```python
from build123d import *

# Parameters (mm, degrees)
SKETCH1_W               = 212.5
SKETCH1_H               = 339.725
BOSS_EXTRUDE1_DEPTH     = 6
SKETCH2_W               = 6.5
SKETCH2_H               = 20
BOSS_EXTRUDE2_DEPTH     = 24
CUT_EXTRUDE1_DEPTH      = 393.36344838
CUT_EXTRUDE1_DEPTH_BACK = 393.36344838
SKETCH3_R               = 4
FILLET2_R               = 5
SKETCH5_R               = 3.175
CUT_EXTRUDE2_DEPTH      = 402.314497153
CUT_EXTRUDE3_DEPTH      = 402.314497153
SKETCH10_R              = 4
CUT_EXTRUDE4_DEPTH      = 18
SKETCH11_R              = 4
CUT_EXTRUDE5_DEPTH      = 14.986


with BuildPart() as part:
    # Sketch1 → Boss-Extrude1 (new body)
    with BuildSketch(Plane.XY):
        with Locations((106.25, -169.8625)):
            Rectangle(SKETCH1_W, SKETCH1_H)
    extrude(amount=BOSS_EXTRUDE1_DEPTH)

    # Sketch2 → Boss-Extrude2 (add)
    with BuildSketch(Plane.XY.offset(6)):
        with Locations((21.75, -35.2425)):
            Rectangle(SKETCH2_W, SKETCH2_H)
        with Locations((50.75, -35.2425)):
            Rectangle(SKETCH2_W, SKETCH2_H)
        with Locations((190.75, -35.2425)):
            Rectangle(SKETCH2_W, SKETCH2_H)
        with Locations((161.75, -35.2425)):
            Rectangle(SKETCH2_W, SKETCH2_H)
        with Locations((133.75, -104.5325)):
            Rectangle(SKETCH2_W, SKETCH2_H)
        with Locations((165.25, -104.5325)):
            Rectangle(SKETCH2_W, SKETCH2_H)
        with Locations((165.25, -235.1925)):
            Rectangle(SKETCH2_W, SKETCH2_H)
        with Locations((21.75, -304.4825)):
            Rectangle(SKETCH2_W, SKETCH2_H)
        with Locations((50.75, -304.4825)):
            Rectangle(SKETCH2_W, SKETCH2_H)
        with Locations((190.75, -304.4825)):
            Rectangle(SKETCH2_W, SKETCH2_H)
        with Locations((161.75, -304.4825)):
            Rectangle(SKETCH2_W, SKETCH2_H)
        with Locations((133.75, -235.1925)):
            Rectangle(SKETCH2_W, SKETCH2_H)
    extrude(amount=BOSS_EXTRUDE2_DEPTH)

    # Sketch3 → Cut-Extrude1 (cut, two sides: drawn at the far end of the back side and taken through both)
    with BuildSketch(Plane.ZY.offset(-18.5).offset(-CUT_EXTRUDE1_DEPTH_BACK)):
        with Locations(Location((18, -35.2425, 0), (0, 0, 180))):
            Circle(SKETCH3_R)
        with Locations((18, -235.1925)):
            Circle(SKETCH3_R)
        with Locations(Location((18, -304.4825, 0), (0, 0, 270))):
            Circle(SKETCH3_R)
        with Locations(Location((18, -104.5325, 0), (0, 0, 180))):
            Circle(SKETCH3_R)
        with BuildLine():
            Line((18, -25.2425), (18, -12.982943413))
            Line((18, -12.982943413), (51.949532367, -12.982943413))
            Line((51.949532367, -12.982943413), (51.949532367, -57.481006387))
            Line((51.949532367, -57.481006387), (18, -57.481006387))
            Line((18, -57.481006387), (18, -45.2425))
            ThreePointArc((18, -45.2425), (28, -35.2425), (18, -25.2425))
        make_face()
        with BuildLine():
            Line((52.442304634, -132.399123951), (18, -132.399123951))
            Line((18, -132.399123951), (18, -114.5325))
            ThreePointArc((18, -114.5325), (28, -104.5325), (18, -94.5325))
            Line((18, -94.5325), (18, -71.59149594))
            Line((18, -71.59149594), (52.442304634, -71.59149594))
            Line((52.442304634, -71.59149594), (52.442304634, -132.399123951))
        make_face()
        with BuildLine():
            Line((52.599532243, -270.375386727), (18, -270.375386727))
            Line((18, -270.375386727), (18, -245.1925))
            ThreePointArc((18, -245.1925), (28, -235.1925), (18, -225.1925))
            Line((18, -225.1925), (18, -207.306351849))
            Line((18, -207.306351849), (52.599532243, -207.306351849))
            Line((52.599532243, -207.306351849), (52.599532243, -270.375386727))
        make_face()
        with BuildLine():
            Line((52.621034016, -326.721115515), (18, -326.721115515))
            Line((18, -326.721115515), (18, -314.4825))
            ThreePointArc((18, -314.4825), (28, -304.4825), (18, -294.4825))
            Line((18, -294.4825), (18, -282.222834285))
            Line((18, -282.222834285), (52.621034016, -282.222834285))
            Line((52.621034016, -282.222834285), (52.621034016, -326.721115515))
        make_face()
    extrude(amount=CUT_EXTRUDE1_DEPTH + CUT_EXTRUDE1_DEPTH_BACK, mode=Mode.SUBTRACT)

    # Fillet2
    fillet2_edges = [part.edges().sort_by_distance(p)[0] for p in [
        (190.75, -45.2425, 6),
        (194, -35.2425, 6),
        (190.75, -25.2425, 6),
        (50.75, -45.2425, 6),
        (54, -35.2425, 6),
        (50.75, -25.2425, 6),
        (21.75, -25.2425, 6),
        (18.5, -35.2425, 6),
        (21.75, -45.2425, 6),
        (161.75, -25.2425, 6),
        (158.5, -35.2425, 6),
        (161.75, -45.2425, 6),
        (161.75, -294.4825, 6),
        (161.75, -314.4825, 6),
        (158.5, -304.4825, 6),
        (190.75, -314.4825, 6),
        (194, -304.4825, 6),
        (190.75, -294.4825, 6),
        (165.25, -245.1925, 6),
        (168.5, -235.1925, 6),
        (165.25, -225.1925, 6),
        (133.75, -225.1925, 6),
        (130.5, -235.1925, 6),
        (133.75, -245.1925, 6),
        (50.75, -314.4825, 6),
        (54, -304.4825, 6),
        (50.75, -294.4825, 6),
        (21.75, -294.4825, 6),
        (21.75, -314.4825, 6),
        (18.5, -304.4825, 6),
        (165.25, -114.5325, 6),
        (165.25, -94.5325, 6),
        (168.5, -104.5325, 6),
        (133.75, -94.5325, 6),
        (130.5, -104.5325, 6),
        (133.75, -114.5325, 6),
    ]]
    fillet(fillet2_edges, radius=FILLET2_R)

    # Sketch5 → Cut-Extrude2 (cut, through all)
    with BuildSketch(Plane.XY.offset(6)):
        with Locations((12.7, -12.7)):
            Circle(SKETCH5_R)
        with Locations((199.8, -12.7)):
            Circle(SKETCH5_R)
        with Locations((66.25, -35.2425)):
            Circle(SKETCH5_R)
        with Locations((146.25, -35.2425)):
            Circle(SKETCH5_R)
        with Locations((176.25, -57.8625)):
            Circle(SKETCH5_R)
        with Locations((36.25, -57.8625)):
            Circle(SKETCH5_R)
        with Locations((191.25, -104.5325)):
            Circle(SKETCH5_R)
        with Locations((36.25, -169.8625)):
            Circle(SKETCH5_R)
        with Locations((191.25, -169.8625)):
            Circle(SKETCH5_R)
        with Locations((36.25, -281.8625)):
            Circle(SKETCH5_R)
        with Locations((66.25, -304.4825)):
            Circle(SKETCH5_R)
        with Locations((12.7, -327.025)):
            Circle(SKETCH5_R)
        with Locations((199.8, -327.025)):
            Circle(SKETCH5_R)
        with Locations((146.25, -304.4825)):
            Circle(SKETCH5_R)
        with Locations(Location((191.25, -235.1925, 0), (0, 0, 180))):
            Circle(SKETCH5_R)
    extrude(amount=-CUT_EXTRUDE2_DEPTH, mode=Mode.SUBTRACT)

    # Sketch9 → Cut-Extrude3 (cut, through all)
    with BuildSketch(Plane.XY.offset(6)):
        with BuildLine():
            Line((70, -271.3625), (110, -271.3625))
            ThreePointArc((110, -271.3625), (114.242640687, -269.605140687), (116, -265.3625))
            Line((116, -265.3625), (116, -74.3625))
            ThreePointArc((116, -74.3625), (114.242640687, -70.119859313), (110, -68.3625))
            Line((110, -68.3625), (70, -68.3625))
            ThreePointArc((70, -68.3625), (65.757359313, -70.119859313), (64, -74.3625))
            Line((64, -74.3625), (64, -265.3625))
            ThreePointArc((64, -265.3625), (65.757359313, -269.605140687), (70, -271.3625))
        make_face()
    extrude(amount=-CUT_EXTRUDE3_DEPTH, mode=Mode.SUBTRACT)

    # Sketch10 → Cut-Extrude4 (cut)
    with BuildSketch(Plane.XY.offset(6)):
        with Locations((76.95, -316.111459893)):
            Circle(SKETCH10_R)
    extrude(amount=-CUT_EXTRUDE4_DEPTH, mode=Mode.SUBTRACT)

    # Sketch11 → Cut-Extrude5 (cut)
    with BuildSketch(Plane.XY.offset(6)):
        with Locations((76.9625, -23.613540107)):
            Circle(SKETCH11_R)
    extrude(amount=-CUT_EXTRUDE5_DEPTH, mode=Mode.SUBTRACT)


solid = part.part
```
Read the model definition and answer for the solid it produces. Units are mm, in the model's axes. A direction names the side the tool comes from. Coordinates: 2 decimals unless noted, no trailing zeros. Write each loop counter-clockwise with the first axis right and the second up, starting at its lowest first coordinate (ties: lowest second). Pieces come first, ordered by that corner, then holes. Notation, with made-up numbers: (16, 83.25) -> (27, 83.25) arc R14 cw to (27, 96.25) -> close; hole circle Ø5 at (-4.5, 46). An arc over 180 degrees is marked (long way). Answer as a JSON object with one key per item and string values.
Q1. The part is cut by section B-B on y = -84. Give the vertices of the cut face in (x, z), then the cut area to 3 significant figures.
The answers:
{"outline": "(0, 0) -> (64, 0) -> (64, 6) -> (0, 6) -> close; (116, 0) -> (212.5, 0) -> (212.5, 6) -> (116, 6) -> close", "area": "963 mm2"}
Q2. Determine the mould class of faces 4 (the flat face through (54, -31, 19)), 5 (the cylindrical face through (78.81, -27.16, 3.04)), 6 (the flat face through (18.5, -31, 19)), 7 (the cylindrical face through (133.796, -239.097, 17.133)) for opening direction X: pulls with the +X half, pulls with the -X half, needs draft (parallel to the pull), parting line crosses it, or undercut.
The answers:
{"face 4": "undercut", "face 5": "undercut", "face 6": "pulls with the -X half", "face 7": "needs draft"}
Q3. The part is cut by section A-A on x = 87. Give the vertices of the cut face in (y, z) (1 decimal), then the cut area to 3 significant figures.
The answers:
{"outline": "(-339.7, 0) -> (-271.4, 0) -> (-271.4, 6) -> (-339.7, 6) -> close; (-68.4, 0) -> (0, 0) -> (0, 6) -> (-68.4, 6) -> close", "area": "820 mm2"}
Q4. Consider line 1 (Y direction, x = 199.8, z = 2.25) (3 decimals); line 2 (X direction, y = -35.5, z = 2); line 3 (X direction, y = -312.5, z = 22). Determine where each line is inside the solid, lowest interval first. Write a range as [from, to].
The answers:
{"line 1": "y = [-339.725, -330.2], [-323.85, -15.875], [-9.525, 0]", "line 2": "x = [0, 63.09], [69.41, 143.09], [149.41, 212.5]", "line 3": "x = [18.5, 25], [47.5, 54], [158.5, 165], [187.5, 194]"}
Q5. A tool of negligible diameter and unlimited length cuts with its end or side. For faces 1 (the flat face through (137, -101, 14)), 2 (the flat face through (51, -294.482, 14)), 3 (the flat face through (162, -101, 14)), from which of +Z, -Z, +X, -X, +Y, -Y can it reach the whole face along a straight path? Write none if from no direction.
The answers:
{"face 1": "+Z, +Y, -Y", "face 2": "+Z, +X, -X", "face 3": "+Z"}
Q6. Flat-ended cylindrical pins translate along their axes: pin 1 Ø7 at (x, z) = (22.5, 13) entering from +Y; pin 2 Ø3 at (x, z) = (160.5, 15) entering from -Y; pin 3 Ø7 at (x, z) = (164, 14.5) entering from +Y. Find the tip coordinate at first contact, or state that the pin passes through.
The answers:
{"pin 1": "stops at y = -25.01", "pin 2": "stops at y = -314.48", "pin 3": "stops at y = -25.24"}
